Source: CAD feature listing. Evaluate the final solid. Frame: model axes, mm. A direction names the side the tool comes from. Give positions to 0.01 mm unless a question says otherwise; leave off trailing zeros. Write each loop counter-clockwise with the first axis right and the second up, starting at its lowest first coordinate (ties: lowest second). Pieces come first, ordered by that corner, then holes. Notation, with made-up numbers: (48.25, 18.5) - (97.25, 18.5) arc R18 ccw to (97.25, 26.5) - close; hole circle Ø7 at (32, 4.5). An arc over 180 degrees is marked (long way). One line per question, with ' | ' between items. Start each with the question number.
(1) Section D-D, the plane y = 42. Return loops of the section in (x, z), plus the area to 3 significant figures.
(2) Section A-A, the plane x = -24. Return loops of the section in (y, z).
(3) Ray query, line 1 (X direction, y = -15, z = 6); line 2 (X direction, y = -5.5, z = 5.25); line 3 (Y direction, x = -35.5, z = 1.75). Return the intervals inside material, ascending. Write a range as [from, to].
(4) Section B-B, the plane z = 5.25. Return loops of the section in (x, y), plus the area to 3 significant figures.
(5) Section C-C, the plane y = 14. Return loops of the section in (x, z).
(6) Access query for faces 1 (the flat face through (5.09, 35.27, 12.87)), 2 (the flat face through (-11.24, 56.08, 13.69)), 3 (the flat face through (4.62, -8.56, 12.48)). Directions: +Z, -Z, +X, -X, +Y, -Y. A direction counts if a zero-diameter tool reaches every point of the face in a straight line with its end or side. Return the directions, or none.
(7) Draft query along Y for faces 4 (the flat face through (-44.93, 49.784, 13.425)), 5 (the flat face through (-26.19, -26.74, 13.43)), 6 (the flat face through (-31.454, -21.511, 12.477)). Return one class per face: +Y half, -Y half, draft (parallel to the pull), parting line (faces both ways), or undercut.
(8) Pin query (flat end, axial travel): pin 1 (6 mm diameter, centred on y = 18.5, z = 7.5, fed in from -X); pin 2 (4.5 mm diameter, centred on x = 7.5, y = 25, fed in from +Z); pin 3 (4.5 mm diameter, centred on x = -35, y = -13, fed in from +Z). Return the tip coordinate at first contact, or that it passes through.
```python
from build123d import *

# Parameters (mm, degrees)
BOSS_EXTRUDE3_DEPTH = 14.43945182
BOSS_EXTRUDE4_DEPTH = 1.453195813
SKETCH3_W           = 39
SKETCH3_H           = 11.33945182
CUT_EXTRUDE2_DEPTH  = 20
SKETCH6_W           = 20
SKETCH6_H           = 3.175
CUT_EXTRUDE3_DEPTH  = 20
SKETCH5_W           = 20
SKETCH5_H           = 3.175
CUT_EXTRUDE4_DEPTH  = 20
SKETCH8_W           = 3.175
SKETCH8_H           = 20
CUT_EXTRUDE5_DEPTH  = 20
SKETCH7_W           = 3.175
SKETCH7_H           = 20
CUT_EXTRUDE6_DEPTH  = 20
CHAMFER1_SIZE       = 2
CHAMFER2_SIZE       = 2


with BuildPart() as part:
    # Sketch1 → Boss-Extrude3 (new body)
    with BuildSketch(Plane.XY):
        Polygon((-59.137511347, -0.038105162), (-21.037511347, -32.416956285), (17.062488653, -0.038105162), (0.174311479, 63.764633586), (-42.249334174, 63.764633586), align=None)
        Polygon((-21.037511347, -29.017601836), (-55.137511347, -0.038105162), (-40.729968911, 52.414123882), (-21.037511347, 59.708444624), (-1.345053783, 52.414123882), (13.062488653, -0.038105162), align=None, mode=Mode.SUBTRACT)
    extrude(amount=BOSS_EXTRUDE3_DEPTH)

    # Sketch1<5> → Boss-Extrude4 (add)
    with BuildSketch(Plane.XY):
        Polygon((-55.137511347, -0.038105162), (-40.729968911, 52.414123882), (-21.037511347, 59.708444624), (-1.345053783, 52.414123882), (13.062488653, -0.038105162), (-21.037511347, -29.017601836), align=None)
    extrude(amount=BOSS_EXTRUDE4_DEPTH)

    # Sketch3 → Cut-Extrude2 (cut)
    with BuildSketch(Plane(origin=(0, 63.764633586, 0), x_dir=(1, 0, 0), z_dir=(0, 1, 0))):
        with Locations((-21.039334174, -7.76972591)):
            Rectangle(SKETCH3_W, SKETCH3_H)
    extrude(amount=-CUT_EXTRUDE2_DEPTH, mode=Mode.SUBTRACT)

    # Sketch6 → Cut-Extrude3 (cut)
    with BuildSketch(Plane(origin=(7.174060124, -8.441673539, 0), x_dir=(0.762, 0.6475770224459791, 0), z_dir=(0.647577022445979, -0.7619999999999999, 0))):
        with Locations((-12.023059674, 12.85195182)):
            Rectangle(SKETCH6_W, SKETCH6_H)
    extrude(amount=-CUT_EXTRUDE3_DEPTH, mode=Mode.SUBTRACT)

    # Sketch5 → Cut-Extrude4 (cut)
    with BuildSketch(Plane(origin=(-24.818473342, -29.203748791, 0), x_dir=(0.762, -0.6475770224459791, 0), z_dir=(-0.647577022445979, -0.7619999999999999, 0))):
        with Locations((-20.038107619, 12.85195182)):
            Rectangle(SKETCH5_W, SKETCH5_H)
    extrude(amount=-CUT_EXTRUDE4_DEPTH, mode=Mode.SUBTRACT)

    # Sketch8 → Cut-Extrude5 (cut)
    with BuildSketch(Plane(origin=(15.935890818, 4.218128451, 0), x_dir=(0, 0, -1), z_dir=(0.9667081628497367, 0.2558814723259324, 0))):
        with Locations((-12.85195182, 22.79218871)):
            Rectangle(SKETCH8_W, SKETCH8_H)
    extrude(amount=-CUT_EXTRUDE5_DEPTH, mode=Mode.SUBTRACT)

    # Sketch7 → Cut-Extrude6 (cut)
    with BuildSketch(Plane(origin=(-55.256037606, 14.625920004, 0), x_dir=(0, 0, 1), z_dir=(-0.9667081628497369, 0.25588147232593195, 0))):
        with Locations((12.85195182, 12.025969955)):
            Rectangle(SKETCH7_W, SKETCH7_H)
    extrude(amount=-CUT_EXTRUDE6_DEPTH, mode=Mode.SUBTRACT)

    # Chamfer1
    # the kernel refuses this chamfer: 2 mm, written as the material it takes off along each edge
    with BuildSketch(Plane(origin=(-53.421537372, 21.556575571, 14.43945182), x_dir=(0.9663426668416519, -0.255784727868533, 0.027495876610586473), z_dir=(-0.255881472325932, -0.9667081628497369, 0))) as chamfer1_piece_1:
        Polygon((CHAMFER1_SIZE * 0.999621916911, -CHAMFER1_SIZE * 0.0274958766106), (-CHAMFER1_SIZE * 0.0274958766106, -CHAMFER1_SIZE * 0.999621916911), (0, 0), align=None)
    extrude(amount=27.481731952, mode=Mode.SUBTRACT)
    with BuildSketch(Plane(origin=(-63.056756221, 3.292620462, 14.43945182), x_dir=(-0.01780569790502669, -0.020951857977268146, -0.9996219169112968), z_dir=(0.762, -0.6475770224459791, 0)), Plane(origin=(-36.386756221, -19.372575324, 14.43945182), x_dir=(-0.017805697905026844, -0.020951857977268323, -0.9996219169112968), z_dir=(0.762, -0.6475770224459791, 0)), Plane(origin=(-24.956756221, -35.747681909, 14.43945182), x_dir=(0.017805697905025137, -0.020951857977266314, -0.9996219169112968), z_dir=(0.762, 0.6475770224459791, 0)), Plane(origin=(1.713243779, -13.082486123, 14.43945182), x_dir=(0.01780569790502548, -0.02095185797726672, -0.9996219169112968), z_dir=(0.762, 0.6475770224459791, 0))) as chamfer1_piece_2:
        Polygon((CHAMFER1_SIZE * 0.999621916911, CHAMFER1_SIZE * 0.0274958766106), (-CHAMFER1_SIZE * 0.0274958766106, CHAMFER1_SIZE * 0.999621916911), (0, 0), align=None)
    extrude(amount=25.286731952, mode=Mode.SUBTRACT)
    with BuildSketch(Plane(origin=(18.378580711, -5.010239036, 14.43945182), x_dir=(0.02658048836416282, 0.007035685390008962, -0.9996219169112968), z_dir=(-0.2558814723259324, 0.9667081628497367, 0))) as chamfer1_piece_3:
        Polygon((CHAMFER1_SIZE * 0.999621916911, CHAMFER1_SIZE * 0.0274958766106), (-CHAMFER1_SIZE * 0.0274958766106, CHAMFER1_SIZE * 0.999621916911), (0, 0), align=None)
    extrude(amount=27.481731952, mode=Mode.SUBTRACT)
    with BuildSketch(Plane(origin=(8.861069348, 30.946471081, 14.43945182), x_dir=(0.026580488364163036, 0.007035685390009019, -0.9996219169112968), z_dir=(-0.2558814723259324, 0.9667081628497367, 0)), Plane(origin=(-40.933242115, 68.736767459, 14.43945182), x_dir=(-0.026580488364161756, 0.007035685390008668, -0.9996219169112968), z_dir=(-0.255881472325932, -0.9667081628497369, 0))) as chamfer1_piece_4:
        Polygon((CHAMFER1_SIZE * 0.999621916911, CHAMFER1_SIZE * 0.0274958766106), (-CHAMFER1_SIZE * 0.0274958766106, CHAMFER1_SIZE * 0.999621916911), (0, 0), align=None)
    extrude(amount=39.091731952, mode=Mode.SUBTRACT)
    with BuildSketch(Plane(origin=(5.317677455, 63.764633586, 14.43945182), x_dir=(0, 0.027495876610585623, -0.9996219169112968), z_dir=(-1, 0, 0))) as chamfer1_piece_5:
        Polygon((CHAMFER1_SIZE * 0.999621916911, CHAMFER1_SIZE * 0.0274958766106), (-CHAMFER1_SIZE * 0.0274958766106, CHAMFER1_SIZE * 0.999621916911), (0, 0), align=None)
    extrude(amount=52.710377605, mode=Mode.SUBTRACT)

    # Chamfer2
    chamfer2_edges = [part.edges().sort_by_distance(p)[0] for p in [
        (-50.693422761, 31.863264212, 0),
        (8.618400066, 31.863264212, 0),
        (-1.987511347, -16.227530724, 0),
        (-40.087511347, -16.227530724, 0),
    ]]
    chamfer(chamfer2_edges, length=CHAMFER2_SIZE)


solid = part.part
```
Check sheet entries:
1) outline: (-48.01, 2) - (-45.94, 0) - (3.87, 0) - (5.94, 2) - (5.94, 12.44) - (3.87, 14.44) - (1.52, 14.44) - (1.52, 1.45) - (-43.59, 1.45) - (-43.59, 14.44) - (-45.94, 14.44) - (-48.01, 12.44) - close | area: 185 mm²
2) outline: (-29.9, 2) - (-27.27, 0) - (63.76, 0) - (63.76, 2.1) - (58.61, 2.1) - (58.61, 1.45) - (-26.5, 1.45) - (-26.5, 14.44) - (-27.27, 14.44) - (-29.9, 12.44) - close; (58.61, 13.44) - (62.76, 13.44) - (61.76, 14.44) - (58.61, 14.44) - close
3) line 1: [-41.53, -37.53], [-4.54, -0.54] | line 2: [-52.71, -48.71], [6.64, 10.64] | line 3: [-19.8, -16.73], [54.35, 63.76]
4) outline: (-59.14, -0.04) - (-21.04, -32.42) - (17.06, -0.04) - (0.17, 63.76) - (-1.54, 63.76) - (-1.54, 52.49) - (-1.35, 52.41) - (13.06, -0.04) - (-21.04, -29.02) - (-55.14, -0.04) - (-40.73, 52.41) - (-40.54, 52.48) - (-40.54, 63.76) - (-42.25, 63.76) - close | area: 765 mm²
5) outline: (-55.42, 2) - (-53.35, 0) - (11.28, 0) - (13.35, 2) - (13.35, 12.44) - (11.28, 14.44) - (9.21, 14.44) - (9.21, 1.45) - (-51.28, 1.45) - (-51.28, 14.44) - (-53.35, 14.44) - (-55.42, 12.44) - close
6) face 1: +Z, +X | face 2: +Z | face 3: +Z, -Y
7) face 4: +Y half | face 5: -Y half | face 6: undercut
8) pin 1: x = -55.02 | pin 2: z = 11.26 | pin 3: z = 1.45
